Input: part model. Units: mm. Frame: model coordinates. A direction names the side the tool comes from. Give positions to 0.01 mm unless a question says otherwise; leave off trailing zeros. Loops run counter-clockwise (first coordinate to the right, second up) from the corner with the lowest first, then second, coordinate; pieces in that order, holes last. Notation, with made-up numbers: (-13.5, -8.5) -> (43.5, -8.5) arc R23 ccw to (43.5, 9.5) -> close; hole circle Ø11 at (13, 33). An arc over 180 degrees is marked (long way). Answer as a JSON object with one key per item and string values.
```python
from build123d import *

# Parameters (mm, degrees)
SKETCH1_R           = 5
BOSS_EXTRUDE1_DEPTH = 30.5
SKETCH24_R          = 5
SKETCH24_R_2        = 4.5
CUT_EXTRUDE3_DEPTH  = 2.5
SKETCH25_R          = 5
SKETCH25_R_2        = 4.5
CUT_EXTRUDE4_DEPTH  = 2.5


with BuildPart() as part:
    # Sketch1 → Boss-Extrude1 (new body)
    with BuildSketch(Plane(origin=(0, 0, 0), x_dir=(1, 0, 0), z_dir=(0, 1, 0))):
        Circle(SKETCH1_R)
    extrude(amount=BOSS_EXTRUDE1_DEPTH)

    # Sketch24 → Cut-Extrude3 (cut)
    with BuildSketch(Plane(origin=(0, 0, 0), x_dir=(-1, 0, 0), z_dir=(0, -1, 0))):
        Circle(SKETCH24_R)
        Circle(SKETCH24_R_2, mode=Mode.SUBTRACT)
    extrude(amount=-CUT_EXTRUDE3_DEPTH, mode=Mode.SUBTRACT)

    # Sketch25 → Cut-Extrude4 (cut)
    with BuildSketch(Plane(origin=(0, 30.5, 0), x_dir=(1, 0, 0), z_dir=(0, 1, 0))):
        Circle(SKETCH25_R)
        Circle(SKETCH25_R_2, mode=Mode.SUBTRACT)
    extrude(amount=-CUT_EXTRUDE4_DEPTH, mode=Mode.SUBTRACT)


solid = part.part
```
Q1. Section D-D, the plane y = 28.5. Return the cut outline in (x, z).
Evaluation:
{"outline": "circle Ø9 at (0, 0)"}
Q2. Section A-A, the plane x = 0. Return the cut outline in (y, z), then the cut area to 3 significant figures.
Evaluation:
{"outline": "(0, -4.5) -> (2.5, -4.5) -> (2.5, -5) -> (28, -5) -> (28, -4.5) -> (30.5, -4.5) -> (30.5, 4.5) -> (28, 4.5) -> (28, 5) -> (2.5, 5) -> (2.5, 4.5) -> (0, 4.5) -> close", "area": "300 mm2"}
Q3. Pin query (flat end, axial travel): pin 1 (2 mm diameter, centred on y = 13.5, z = -4, fed in from -X); pin 2 (2 mm diameter, centred on x = 3.5, y = 12, fed in from +Z); pin 3 (4 mm diameter, centred on y = 10, z = -3.5, fed in from +X). Return the tip coordinate at first contact, or that it passes through.
Evaluation:
{"pin 1": "stops at x = -4", "pin 2": "stops at z = 4.33", "pin 3": "stops at x = 4.77"}
Q4. Access query for faces 1 (the cylindrical face through (0.59, 1.23, -4.46)), 2 (the cylindrical face through (-1.08, 15.07, 4.88)), 3 (the cylindrical face through (-0.59, 29.27, -4.46)). Directions: +Z, -Z, +X, -X, +Y, -Y. A direction counts if a zero-diameter tool reaches every point of the face in a straight line with its end or side. Return the directions, or none.
Evaluation:
{"face 1": "-Y", "face 2": "+Y, -Y", "face 3": "+Y"}
Q5. Section B-B, the plane z = 0. Return the cut outline in (x, y), then the cut area to 3 significant figures.
Evaluation:
{"outline": "(-5, 2.5) -> (-4.5, 2.5) -> (-4.5, 0) -> (4.5, 0) -> (4.5, 2.5) -> (5, 2.5) -> (5, 28) -> (4.5, 28) -> (4.5, 30.5) -> (-4.5, 30.5) -> (-4.5, 28) -> (-5, 28) -> close", "area": "300 mm2"}
Q6. Ray query, line 1 along Z through (x, y) = (0.25, 3); line 2 along Y through (x, z) = (-4.25, 2.25); line 3 along Z through (x, y) = (-0.75, 14.5). Return the intervals inside material, ascending.
Evaluation:
{"line 1": "z = -4.99 to 4.99", "line 2": "y = 2.5 to 28", "line 3": "z = -4.94 to 4.94"}
Q7. Section C-C, the plane y = 4.5. Return the cut outline in (x, z), then the cut area to 3 significant figures.
Evaluation:
{"outline": "circle Ø10 at (0, 0)", "area": "78.5 mm2"}
